```python
from build123d import *

# Parameters (mm, degrees)
SKETCH_1_R          = 7.9
SKETCH_1_R_2        = 5
EXTRUDE_1_DEPTH     = 3
SKETCH_3_R          = 15
CUT_EXTRUDE_2_DEPTH = 4
FILLET_1_R          = 20


with BuildPart() as part:
    # Эскиз1 → Бобышка-Вытянуть1 (new body)
    with BuildSketch(Plane.XY):
        with BuildLine():
            Line((-19.359148134, 5.022288675), (-52.179574067, -121.488855663))
            ThreePointArc((-52.179574067, -121.488855663), (-45.401310581, -133.569869221), (-33.055555556, -127.286710991))
            ThreePointArc((-33.055555556, -127.286710991), (0, -103.790199458), (33.055555556, -127.286710991))
            ThreePointArc((33.055555556, -127.286710991), (45.401310581, -133.569869221), (52.179574067, -121.488855663))
            Line((52.179574067, -121.488855663), (19.359148134, 5.022288675))
            ThreePointArc((19.359148134, 5.022288675), (0, 20), (-19.359148134, 5.022288675))
        make_face()
        Circle(SKETCH_1_R, mode=Mode.SUBTRACT)
        with Locations((-42.5, -124)):
            Circle(SKETCH_1_R_2, mode=Mode.SUBTRACT)
        with Locations((42.5, -124)):
            Circle(SKETCH_1_R_2, mode=Mode.SUBTRACT)
    extrude(amount=EXTRUDE_1_DEPTH)

    # Эскиз3 → Вырез-Вытянуть2 (cut, through all)
    with BuildSketch(Plane.XY.offset(3)):
        with Locations((-38, -56.391488719)):
            Circle(SKETCH_3_R)
        with Locations((38, -56.391488719)):
            Circle(SKETCH_3_R)
    extrude(amount=-CUT_EXTRUDE_2_DEPTH, mode=Mode.SUBTRACT)

    # Скругление1
    fillet_1_edges = [part.edges().sort_by_distance(p)[0] for p in [
        (-39.171079178, -71.345704632, 1.5),
        (-31.7536013, -42.753948498, 1.5),
        (31.7536013, -42.753948498, 1.5),
        (39.171079178, -71.345704632, 1.5),
    ]]
    fillet(fillet_1_edges, radius=FILLET_1_R)


solid = part.part
```
Check sheet for the modelled part. Datum: model origin and axes. Units: mm. Coordinates: 2 decimals unless noted, no trailing zeros. Write each loop counter-clockwise with the first axis right and the second up, starting at its lowest first coordinate (ties: lowest second). Pieces come first, ordered by that corner, then holes. Notation, with made-up numbers: M 87.5,53 L 119.5,53 A3 ccw 119.5,58 Z; hole C 22.25,26.25 d11. An arc over 180 degrees is marked long. Write item = value, one per line. Start each with the question number.
1. Mould release check, pull along Y, two halves, no side actions. Record for faces 1 (the flat face through (-1, -56, 0)), 2 (the cylindrical face through (-47.495, -123.78, 1.479)), 3 (the cylindrical face through (-38.34, -75.32, 1.52)): pulls with the +Y half, pulls with the -Y half, needs draft (parallel to the pull), parting line crosses it, or undercut.
2. Sectioned sample at D-D (x = 11). Record the cut outline in (y, z), then the cut area to 3 significant figures.
3. Sectioned sample at A-A (x = 0). Record the cut outline in (y, z).
4. Thickness scan on probe 1 along Y at (x, z) = (0, 2); probe 2 along X at (y, z) = (-1, 2.2); probe 3 along X at (y, z) = (-56, 2.75). Record the ranges inside material, lowest first.
5. Sectioned sample at B-B (z = 0.5). Record the cut outline in (x, y).
6. Sectioned sample at C-C (y = -19.5). Record the cut outline in (x, z).
7. Go/stop test with a flat-tipped pin: pin 1 (9 mm diameter, centred on x = -42.5, y = -124, fed in from +Z). Record where the tip stops, or that it passes through.
The answers:
q1.face_1 = needs draft
q1.face_2 = undercut
q1.face_3 = pulls with the +Y half
q2.outline = M -105.56,0 L 16.7,0 L 16.7,3 L -105.56,3 Z
q2.area = 367 mm²
q3.outline = M -103.79,0 L -7.9,0 L -7.9,3 L -103.79,3 Z; M 7.9,0 L 20,0 L 20,3 L 7.9,3 Z
q4.probe_1 = -103.79 to -7.9, 7.9 to 20
q4.probe_2 = -20.92 to -7.84, 7.84 to 20.92
q4.probe_3 = -23.01 to 23.01
q5.outline = M -52.18,-121.49 A10 ccw -33.06,-127.29 A35 cw 33.06,-127.29 A10 ccw 52.18,-121.49 L 42.17,-82.9 A20 ccw 31.49,-69.91 A15 cw 25.74,-47.75 A20 ccw 28.76,-31.2 L 19.36,5.02 A20 ccw -19.36,5.02 L -28.76,-31.2 A20 ccw -25.74,-47.75 A15 cw -31.49,-69.91 A20 ccw -42.17,-82.9 Z; hole C -42.5,-124 d10; hole C 0,0 d15.8; hole C 42.5,-124 d10
q6.outline = M -25.72,0 L 25.72,0 L 25.72,3 L -25.72,3 Z
q7.pin_1 = through
